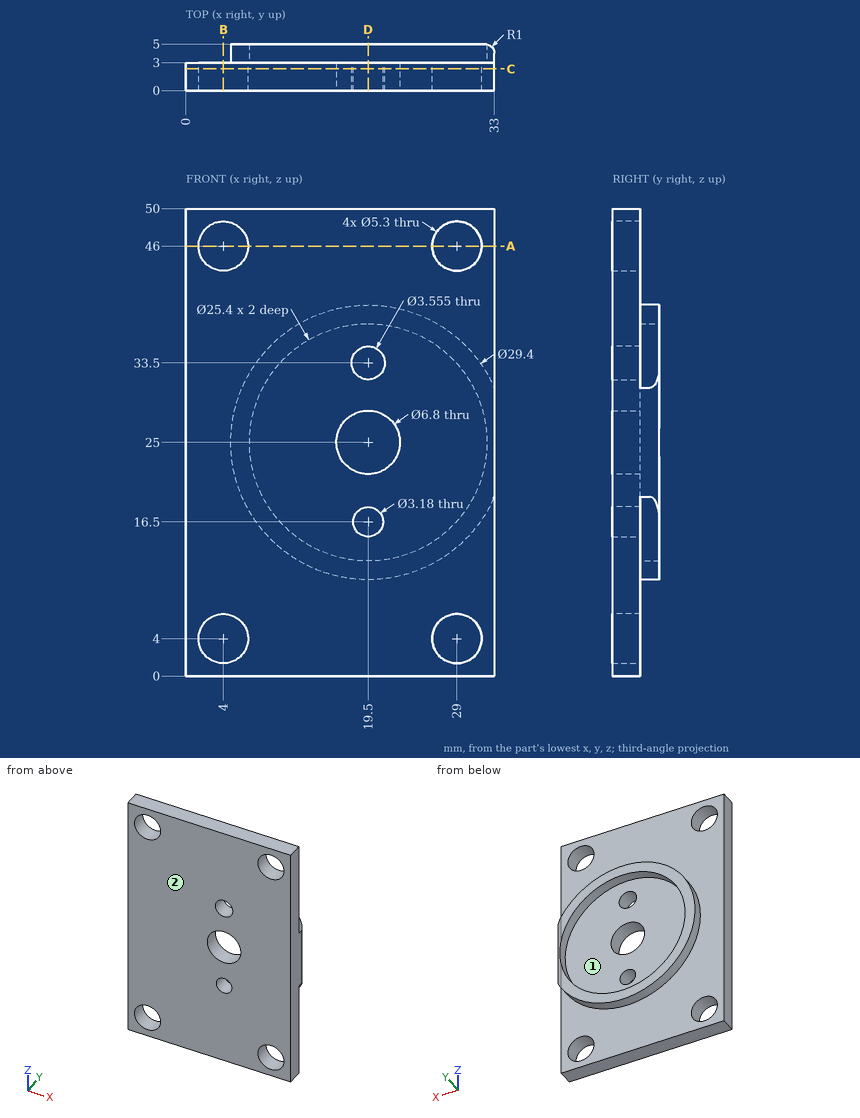
Part print with two shaded views. Sizes in mm from the minimum x, y, z corner. Coordinates: 2 decimals unless noted, no trailing zeros. Write each loop counter-clockwise with the first axis right and the second up, starting at its lowest first coordinate (ties: lowest second). Pieces come first, ordered by that corner, then holes. Notation, with made-up numbers: M 68.25,80.5 L 108.25,80.5 A30 ccw 108.25,117.5 Z; hole C -38,54 d11. An arc over 180 degrees is marked long. Return JSON: item names as keys, results as strings.
Item 1: Drop flat-ended pins along their axis: pin 1 Ø7 at (x, z) = (4, 4) entering from +Y; pin 2 Ø4 at (x, z) = (19.5, 25) entering from -Y. Give the stop position or say it passes through.
Findings below:
{"pin 1": "stops at y = 3", "pin 2": "passes through"}
Item 2: Slice it at D-D, the plane x = 19.5. Write the cut outline in (y, z), and give its area (3 significant figures).
Findings below:
{"outline": "M 0,0 L 3,0 L 3,10.3 L 5,10.3 L 5,12.3 L 3,12.3 L 3,14.91 L 0,14.91 Z; M 0,18.09 L 3,18.09 L 3,21.6 L 0,21.6 Z; M 0,28.4 L 3,28.4 L 3,31.72 L 0,31.72 Z; M 0,35.28 L 3,35.28 L 3,37.7 L 5,37.7 L 5,39.7 L 3,39.7 L 3,50 L 0,50 Z", "area": "117 mm2"}
Item 3: Slice it at C-C, the plane y = 2.35. State how many separate pieces and enclosed holes the cut face has, and give its area (3 significant figures).
Findings below:
{"separate pieces": "1", "enclosed holes": "7", "area": "1,510 mm2"}
Item 4: Slice it at B-B, the plane x = 4. Write the cut outline in (y, z), and give its area (3 significant figures).
Findings below:
{"outline": "M 0,0 L 3,0 L 3,1.35 L 0,1.35 Z; M 0,6.65 L 3,6.65 L 3,43.35 L 0,43.35 Z; M 0,48.65 L 3,48.65 L 3,50 L 0,50 Z", "area": "118 mm2"}
Item 5: Two-plate mould, pull along X, no slides. Class the marked faces 1 and 2: +X half, -X half, draft (parallel to the pull), parting line (faces both ways), or undercut.
Findings below:
{"face 1": "undercut", "face 2": "draft"}
Item 6: Slice it at A-A, the plane z = 46. Write the cut outline in (x, y).
Findings below:
{"outline": "M 0,0 L 1.35,0 L 1.35,3 L 0,3 Z; M 6.65,0 L 26.35,0 L 26.35,3 L 6.65,3 Z; M 31.65,0 L 33,0 L 33,3 L 31.65,3 Z"}
Item 7: Probe line 1 (X direction, y = 1.25, z = 4); line 2 (Z direction, x = 29, y = 2.1); line 3 (Z direction, x = 19.5, y = 3.75). List the from-to ranges inside material, lowest first. Write a range as from..to.
Findings below:
{"line 1": "x = 0..1.35, 6.65..26.35, 31.65..33", "line 2": "z = 0..1.35, 6.65..43.35, 48.65..50", "line 3": "z = 10.3..12.3, 37.7..39.7"}
